Geometry: final body of the model. Coordinates: model frame, mm. A direction names the side the tool comes from. Round coordinates to 2 decimals unless told otherwise and drop trailing zeros. Order: outer loops, then holes, each group sorted by start corner. A loop starts at its lowest first (then second) coordinate and runs counter-clockwise, first axis right, second up. Notation, with made-up numbers: M 25,59 L 30,59 A31 cw 30,86 Z; hole C -23.75,45.25 d8. An arc over 180 degrees is marked long. Put each result on its own line as item: value. Start each with the question number.
1) Section D-D, the plane y = -3.7. Return loops of the section in (x, z), then the cut area to 3 significant figures.
2) Draft query along Y for faces 4 (the flat face through (-54, 2, 7)), 5 (the cylindrical face through (-32.68, -24.61, -1.01)), 6 (the cylindrical face through (51.99, -32.15, -26.99)). Return one class per face: pulls with the +Y half, pulls with the -Y half, needs draft (parallel to the pull), parting line crosses it, or undercut.
3) First-contact query: P1, Ø4, axis at x = 33, y = -0.5, coming from the -Z side; P2, Ø6, axis at x = 6.5, y = -6, coming from the +Z side; P3, Ø9, axis at y = -0.5, z = 5, coming from the +X side. Flat tips, straight axial feed; report the tip coordinate or a pass-through.
4) Section B-B, the plane y = 11.8. Return loops of the section in (x, z), then the cut area to 3 significant figures.
5) Access query for faces 1 (the flat face through (-1, 0, 0)), 2 (the flat face through (51, 0, -17)), 3 (the cylindrical face through (33.21, 7.57, -0.99)). Directions: +Z, -Z, +X, -X, +Y, -Y. A direction counts if a zero-diameter tool reaches every point of the face in a straight line with its end or side. Return the directions, or none.
6) Section A-A, the plane x = 16. Return loops of the section in (y, z), then the cut area to 3 significant figures.
7) Material intervals for probe 1 along Y at (x, z) = (23, -1.15); probe 2 along Z at (x, y) = (-6.5, -21); probe 3 along X at (y, z) = (-12, -27.5), sorted ascending. Write a range as [from, to].
8) Section C-C, the plane x = 38.5. Return loops of the section in (y, z).
from build123d import *

# Parameters (mm, degrees)
SKETCH1_W            = 96
SKETCH1_H            = 70
BASE_FLANGE1_DEPTH   = 2
SKETCH6_R            = 11.05
CUT_EXTRUDE1_DEPTH   = 2
M3_CLEARANCE_HOLE1_D = 3.6
EDGE_FLANGE1_DEPTH   = 67
M5_CLEARANCE_HOLE1_D = 5.8
EDGE_FLANGE2_DEPTH   = 70
FILLET1_R            = 10
FILLET2_R            = 1.5


# Sheet-metal steps are written as plain solids
with BuildPart() as part:
    # Sketch1 → Base-Flange1 (new body)
    with BuildSketch(Plane.XY):
        Rectangle(SKETCH1_W, SKETCH1_H)
    extrude(amount=-BASE_FLANGE1_DEPTH)

    # Sketch6 → Cut-Extrude1 (cut)
    with BuildSketch(Plane.XY):
        with Locations((23, 11.8)):
            Circle(SKETCH6_R)
    extrude(amount=-CUT_EXTRUDE1_DEPTH, mode=Mode.SUBTRACT)

    # M3 Clearance Hole1 (through all)
    with Locations(Plane.XY):
        with Locations((38.5, 27.3), (38.5, -3.7), (7.5, 27.3), (7.5, -3.7)):
            Hole(M3_CLEARANCE_HOLE1_D / 2)

    # Edge-Flange1 section (across the edge) → Edge-Flange1 (add)
    with BuildSketch(Plane(origin=(-52, 35, 0), x_dir=(1, 0, 0), z_dir=(0, -1, 0))):
        with BuildLine():
            Line((-2, 2), (-2, 13))
            Line((-2, 13), (0, 13))
            Line((0, 13), (0, 2))
            ThreePointArc((0, 2), (0.585786438, 0.585786438), (2, 0))
            Line((2, 0), (4, 0))
            Line((4, 0), (4, -2))
            Line((4, -2), (2, -2))
            ThreePointArc((2, -2), (-0.828427125, -0.828427125), (-2, 2))
        make_face()
    extrude(amount=EDGE_FLANGE1_DEPTH)

    # M5 Clearance Hole1 (through all)
    with Locations(Plane.XY):
        with Locations((30, -23.5), (-30, -23.5)):
            Hole(M5_CLEARANCE_HOLE1_D / 2)

    # Edge-Flange2 section (across the edge) → Edge-Flange2 (add)
    with BuildSketch(Plane(origin=(51, 35, -2), x_dir=(-1, 0, 0), z_dir=(0, -1, 0))):
        with BuildLine():
            Line((-2, 2), (-2, 28))
            Line((-2, 28), (0, 28))
            Line((0, 28), (0, 2))
            ThreePointArc((0, 2), (0.585786438, 0.585786438), (2, 0))
            Line((2, 0), (3, 0))
            Line((3, 0), (3, -2))
            Line((3, -2), (2, -2))
            ThreePointArc((2, -2), (-0.828427125, -0.828427125), (-2, 2))
        make_face()
    extrude(amount=EDGE_FLANGE2_DEPTH)

    # Fillet1
    fillet1_edges = [part.edges().sort_by_distance(p)[0] for p in [
        (52, 35, -30),
        (52, -35, -30),
        (-53, 35, 13),
        (-53, -32, 13),
    ]]
    fillet(fillet1_edges, radius=FILLET1_R)

    # Fillet2
    fillet2_edges = [part.edges().sort_by_distance(p)[0] for p in [
        (-48, -32, -1),
    ]]
    fillet(fillet2_edges, radius=FILLET2_R)
    fillet2_2_edges = [part.edges().sort_by_distance(p)[0] for p in [
        (-48, -35, -1),
    ]]
    fillet(fillet2_2_edges, radius=FILLET2_R - 0.0001)  # a hair under: the kernel refuses the full size


solid = part.part
Result sheet:
1. outline: M -54,2 A4 ccw -50,-2 L 5.7,-2 L 5.7,0 L -50,0 A2 cw -52,2 L -52,13 L -54,13 Z; M 9.3,-2 L 36.7,-2 L 36.7,0 L 9.3,0 Z; M 40.3,-2 L 49,-2 A2 cw 51,-4 L 51,-30 L 53,-30 L 53,-4 A4 ccw 49,0 L 40.3,0 Z
1. area: 276 mm2
2. face 4: needs draft
2. face 5: undercut
2. face 6: pulls with the -Y half
3. P1: stops at z = -2
3. P2: stops at z = 0
3. P3: stops at x = -51.32
4. outline: M -54,2 A4 ccw -50,-2 L 11.95,-2 L 11.95,0 L -50,0 A2 cw -52,2 L -52,13 L -54,13 Z; M 34.05,-2 L 49,-2 A2 cw 51,-4 L 51,-30 L 53,-30 L 53,-4 A4 ccw 49,0 L 34.05,0 Z
4. area: 247 mm2
5. face 1: +Z, +X, +Y, -Y
5. face 2: -Z, -X, +Y, -Y
5. face 3: +Z, -Z
6. outline: M -35,-2 L 3.25,-2 L 3.25,0 L -35,0 Z; M 20.35,-2 L 35,-2 L 35,0 L 20.35,0 Z
6. area: 106 mm2
7. probe 1: y = [-35, 0.75], [22.85, 35]
7. probe 2: z = [-2, 0]
7. probe 3: x = [51, 53]
8. outline: M -35,-2 L -5.5,-2 L -5.5,0 L -35,0 Z; M -1.9,-2 L 25.5,-2 L 25.5,0 L -1.9,0 Z; M 29.1,-2 L 35,-2 L 35,0 L 29.1,0 Z
